from build123d import *

# Parameters (mm, degrees)
SKETCH_1_W          = 79
SKETCH_1_H          = 27
EXTRUDE_1_DEPTH     = 10
SKETCH_3_R          = 7.5
CUT_EXTRUDE_1_DEPTH = 43.924352063
SKETCH_4_R          = 5.15
CUT_EXTRUDE_2_DEPTH = 43.924352063
SKETCH_5_R          = 1.75
CUT_EXTRUDE_3_DEPTH = 43.924352063


with BuildPart() as part:
    # 草图1 → 凸台-拉伸1 (new body)
    with BuildSketch(Plane(origin=(0, 0, 0), x_dir=(1, 0, 0), z_dir=(0, 1, 0))):
        Rectangle(SKETCH_1_W, SKETCH_1_H)
    extrude(amount=EXTRUDE_1_DEPTH)

    # 草图3 → 切除-拉伸1 (cut, through all)
    with BuildSketch(Plane(origin=(0, 10, 0), x_dir=(1, 0, 0), z_dir=(0, 1, 0))):
        with Locations(Location((-27, 0, 0), (0, 0, 270))):
            Circle(SKETCH_3_R)
        with Locations(Location((27, 0, 0), (0, 0, 270))):
            Circle(SKETCH_3_R)
    extrude(amount=-CUT_EXTRUDE_1_DEPTH, mode=Mode.SUBTRACT)

    # 草图4 → 切除-拉伸2 (cut, through all)
    with BuildSketch(Plane(origin=(0, 10, 0), x_dir=(1, 0, 0), z_dir=(0, 1, 0))):
        with Locations(Location((0, 0, 0), (0, 0, 270))):
            Circle(SKETCH_4_R)
    extrude(amount=-CUT_EXTRUDE_2_DEPTH, mode=Mode.SUBTRACT)

    # 草图5 → 切除-拉伸3 (cut, through all)
    with BuildSketch(Plane(origin=(0, 10, 0), x_dir=(1, 0, 0), z_dir=(0, 1, 0))):
        with Locations(Location((8, 0, 0), (0, 0, 270))):
            Circle(SKETCH_5_R)
        with Locations(Location((0, -8, 0), (0, 0, 270))):
            Circle(SKETCH_5_R)
        with Locations(Location((-8, 0, 0), (0, 0, 270))):
            Circle(SKETCH_5_R)
        with Locations(Location((0, 8, 0), (0, 0, 270))):
            Circle(SKETCH_5_R)
    extrude(amount=-CUT_EXTRUDE_3_DEPTH, mode=Mode.SUBTRACT)


solid = part.part
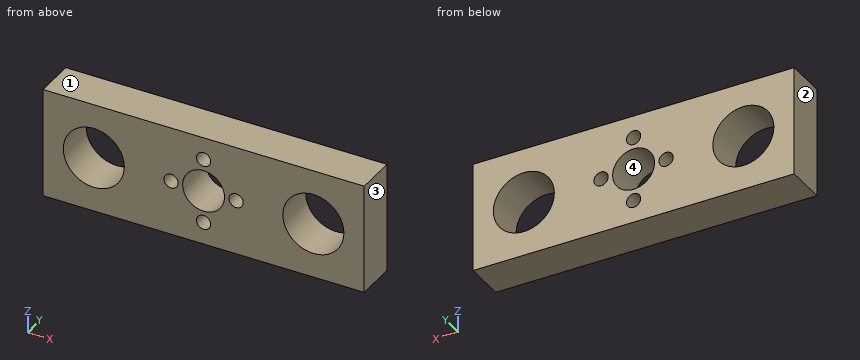
Can you work these out from the model? Positions are in its coordinate system, mm. Face numbers are marked on the shaded views. Round coordinates to 2 decimals unless told otherwise and drop trailing zeros. Loops run counter-clockwise (first coordinate to the right, second up) from the corner with the lowest first, then second, coordinate; pieces in that order, holes last. Notation, with made-up numbers: (84, 21.5) - (106, 21.5) arc R22 ccw to (106, 57.5) - close; hole circle Ø1 at (71, 45). An arc over 180 degrees is marked (long way). Use CSV: the item, a comma, the result in double quotes. Start each with the question number.
1) We'd pull the mould along X, two halves only. Please class the marked faces 1, 2, 3 and 4: released by +X, released by -X, zero draft, split by the parting line, or undercut.
2) If we section it at C-C on x = -27: Write out the boundary of the cut face in (y, z), plus the area to 3 significant figures.
3) If we section it at A-A on x = 8: Write out the boundary of the cut face in (y, z).
4) For pin 1 Ø9 at (x, z) = (-27, 0) entering from -Y; pin 2 Ø5.5 at (x, z) = (0, 8) entering from -Y, each with a flat end and sliding along its axis, tell me the tip position at first contact or that it passes through.
5) If we section it at B-B on y = 5.25: Write out the boundary of the cut face in (x, z), plus the area to 3 significant figures.
6) Please list where these lines run through material, in increasing order: probe 1 along X at (y, z) = (4, 0); probe 2 along X at (y, z) = (5.5, 8); probe 3 along X at (y, z) = (1.25, 3). Write a range as [from, to].
Geometry results:
1,face 1,"zero draft"
1,face 2,"released by -X"
1,face 3,"released by +X"
1,face 4,"undercut"
2,outline,"(0, -13.5) - (10, -13.5) - (10, -7.5) - (0, -7.5) - close; (0, 7.5) - (10, 7.5) - (10, 13.5) - (0, 13.5) - close"
2,area,"120 mm2"
3,outline,"(0, -13.5) - (10, -13.5) - (10, -1.75) - (0, -1.75) - close; (0, 1.75) - (10, 1.75) - (10, 13.5) - (0, 13.5) - close"
4,pin 1,"passes through"
4,pin 2,"stops at y = 0"
5,outline,"(-39.5, -13.5) - (39.5, -13.5) - (39.5, 13.5) - (-39.5, 13.5) - close; hole circle Ø15 at (-27, 0); hole circle Ø3.5 at (-8, 0); hole circle Ø10.3 at (0, 0); hole circle Ø3.5 at (0, -8); hole circle Ø3.5 at (0, 8); hole circle Ø3.5 at (8, 0); hole circle Ø15 at (27, 0)"
5,area,"1,660 mm2"
6,probe 1,"x = [-39.5, -34.5], [-19.5, -9.75], [-6.25, -5.15], [5.15, 6.25], [9.75, 19.5], [34.5, 39.5]"
6,probe 2,"x = [-39.5, -1.75], [1.75, 39.5]"
6,probe 3,"x = [-39.5, -33.87], [-20.13, -4.19], [4.19, 20.13], [33.87, 39.5]"
